Design review of the part built by this model. Coordinates are the model's own, in mm. Face numbers are marked on the shaded views. A direction names the side the tool comes from. Coordinates: 2 decimals unless noted, no trailing zeros. Write each loop counter-clockwise with the first axis right and the second up, starting at its lowest first coordinate (ties: lowest second). Pieces come first, ordered by that corner, then holes. Notation, with made-up numbers: (70.25, 89.5) -> (109.25, 89.5) arc R22 ccw to (109.25, 109.5) -> close; hole circle Ø4 at (-38.5, 67). An arc over 180 degrees is marked (long way). Answer in a Markdown table with one row per item. Add a question column.
Item 1: Clearance check with flat-ended pins moving along their axes: P1, Ø5, axis at x = -3, z = 4.5, coming from the +Y side; P2, Ø3, axis at x = 2, z = 2.5, coming from the +Y side; P3, Ø4, axis at x = 4, y = 7, coming from the -Z side; P4, Ø2.5, axis at x = -1.5, z = 9.5, coming from the -Y side. State where each tip first meets the part, or that it passes through.
Item 2: Take a section at A-A, the plane z = -1. Write out the cut boundary in (x, y).
Item 3: For the marked faces 1, 2 and 3, list the 3-axis set-ups (+Z, -Z, +X, -X, +Y, -Y) from which the entire face can be reached by the end or side of a thin tool; tool diameter is ignored.
Item 4: Take a section at C-C, the plane y = 2.5. Write out the cut boundary in (x, z), and give its area (4 significant figures).
Item 5: Take a section at B-B, the plane x = 0.75. Write out the cut boundary in (y, z), and give its area (3 significant figures).
Item 6: Take a section at D-D, the plane x = 3. Write out the cut boundary in (y, z), and give its area (3 significant figures).
Item 7: To check wall thickness, follow line 1 (Z direction, x = 1, y = 21.75); line 2 (Y direction, x = 4.75, z = -4); line 3 (Y direction, x = 3.75, z = -17.5). State the ranges of each line that lie inside material, in increasing order.
Autodesk Inventor part; units mm, degrees
ref_plane "作業平面1" through (0, 15.4, 0) normal (0, -1, 0) x (1, 0, 0)
ref_plane "YZ Plane" through (0, 0, 0) normal (1, 0, 0) x (0, 1, 0)
ref_plane "XZ Plane" through (0, 0, 0) normal (0, 1, 0) x (-1, 0, 0)
sketch "スケッチ1" plane through (0, 0, 0) normal (0, 1, 0) x (-1, 0, 0)
  line L0 (6.25, -16.75) -> (-6.25, -16.75)
  line L1 (-6.25, -16.75) -> (-6.25, 6.25)
  line L2 (-6.25, 6.25) -> (6.25, 6.25)
  line L3 (6.25, 6.25) -> (6.25, -16.75)
  line L4 (6.25, -16.75) -> (-6.25, 6.25) construction
  line L5 (-6.25, -16.75) -> (6.25, 6.25) construction
  point P0 (0, 0)
  point P1 (0, -5.25)
  dimension "d0" = 12.5
  dimension "d1" = 23
  dimension "d2" = 6.25
extrude "押し出し1" add sketch "スケッチ1" along normal blind 22.6
sketch "スケッチ2" plane through (0, 22.6, 0) normal (0, 1, 0) x (1, 0, 0)
  circle A0 centre (0, 0) radius 6.25
  line L0 (-6.25, -6.25) -> (6.25, -6.25)
  line L1 (6.25, -6.25) -> (6.25, 16.75)
  line L2 (-6.25, 16.75) -> (-6.25, -6.25)
  circle A1 centre (0, 5.65) radius 2.5
  line L3 (-1.87, 7.3093) -> (-4.6749, 4.1482)
  line L4 (1.87, 7.3093) -> (4.6749, 4.1482)
  point P0 (0, 0)
  point P1 (-2.4988, 5.7288)
  point P2 (2.4988, 5.7288)
  dimension "d14" = 5
  dimension "d33" = 11.9
extrude "押し出し2" add sketch "スケッチ2" along normal blind 4.4 contours A0 A1 | A0 A1 L4 | A1 A0 | A0 A1 | A0 L3 A1
ref_plane "作業平面1" through (0, 15.4, 0) normal (0, -1, 0) x (1, 0, 0)
sketch "スケッチ3" plane through (0, 15.4, 0) normal (0, -1, 0) x (1, 0, 0)
  line L0 (-6.25, 11) -> (6.25, 11)
  line L1 (6.25, 11) -> (6.25, -21.5)
  line L2 (6.25, -21.5) -> (-6.25, -21.5)
  line L3 (-6.25, -21.5) -> (-6.25, 11)
  line L4 (-6.25, 11) -> (6.25, -21.5) construction
  line L5 (6.25, 11) -> (-6.25, -21.5) construction
  line L6 (-6.25, 0) -> (-6.25, 6.25)
  line L7 (6.25, 0) -> (6.25, -16.75)
  line L8 (-6.25, -16.75) -> (-6.25, 6.25)
  point P0 (0, 0)
  point P1 (0, -5.25)
  point P2 (-6.25, -5.25)
  dimension "d8" = 32.5
extrude "押し出し3" add sketch "スケッチ3" against normal blind 2.4
sketch "スケッチ4" plane through (0, 27, 0) normal (0, 1, 0) x (1, 0, 0)
  circle A0 centre (0, 0) radius 2.5
  point P0 (0, 0)
  dimension "d11" = 5
extrude "押し出し4" add sketch "スケッチ4" along normal blind 3
properties part number "sg90_Tower_Pro"
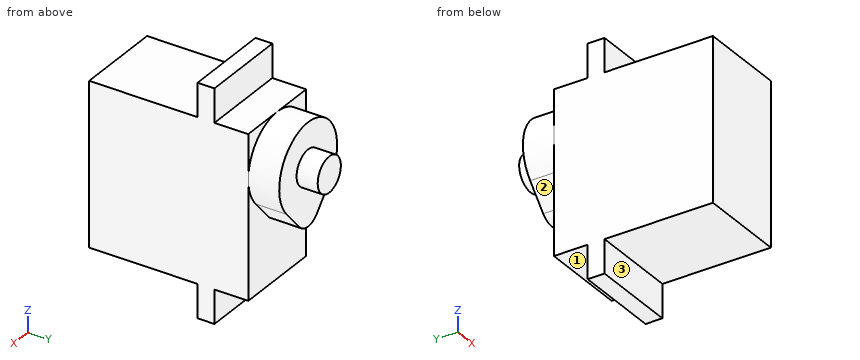
Answers:
| question | item | result |
|---|---|---|
| 1 | P1 | stops at y = 27 |
| 1 | P2 | stops at y = 30 |
| 1 | P3 | stops at z = -16.75 |
| 1 | P4 | stops at y = 15.4 |
| 2 | outline | (-6.25, 0) -> (6.25, 0) -> (6.25, 22.6) -> (6.17, 22.6) -> (6.17, 27) -> (2.29, 27) -> (2.29, 30) -> (-2.29, 30) -> (-2.29, 27) -> (-6.17, 27) -> (-6.17, 22.6) -> (-6.25, 22.6) -> close |
| 3 | face 1 | -Z, +X, -X, +Y |
| 3 | face 2 | -Z, -X, +Y |
| 3 | face 3 | -Z, +X, -X, -Y |
| 4 | outline | (-6.25, -16.75) -> (6.25, -16.75) -> (6.25, 6.25) -> (-6.25, 6.25) -> close |
| 4 | area | 287.5 mm^2 |
| 5 | outline | (0, -16.75) -> (15.4, -16.75) -> (15.4, -21.5) -> (17.8, -21.5) -> (17.8, -16.75) -> (22.6, -16.75) -> (22.6, -8.03) -> (27, -8.03) -> (27, -2.38) -> (30, -2.38) -> (30, 2.38) -> (27, 2.38) -> (27, 6.2) -> (22.6, 6.2) -> (22.6, 6.25) -> (17.8, 6.25) -> (17.8, 11) -> (15.4, 11) -> (15.4, 6.25) -> (0, 6.25) -> close |
| 5 | area | 620 mm^2 |
| 6 | outline | (0, -16.75) -> (15.4, -16.75) -> (15.4, -21.5) -> (17.8, -21.5) -> (17.8, -16.75) -> (22.6, -16.75) -> (22.6, -6.04) -> (27, -6.04) -> (27, 5.48) -> (22.6, 5.48) -> (22.6, 6.25) -> (17.8, 6.25) -> (17.8, 11) -> (15.4, 11) -> (15.4, 6.25) -> (0, 6.25) -> close |
| 6 | area | 593 mm^2 |
| 7 | line 1 | z = -16.75 to 6.25 |
| 7 | line 2 | y = 0 to 27 |
| 7 | line 3 | y = 15.4 to 17.8 |
